Answer from the drawing. Dimensions are ordinates in mm from the lowest x, y and z of the part. A direction names the side the tool comes from. Coordinates: 2 decimals unless noted, no trailing zeros. Write each loop counter-clockwise with the first axis right and the second up, starting at its lowest first coordinate (ties: lowest second). Pieces come first, ordered by that corner, then holes.
(1) The part is cut by section A-A on x = 3. Determine the outline of the cut face in (y, z), plus the area to 3 significant figures.
(2) Which of the six approach directions +Z, -Z, +X, -X, +Y, -Y give full straight-line access (tool end or side, diameter ignored) to the marked faces 4, 5 and 6?
(3) The part is cut by section D-D on y = 5.5. Determine the outline of the cut face in (x, z), plus the area to 3 significant figures.
(4) For a pull along Z with two mould halves and no side action, classify the marked faces 1, 2 and 3 as +Z half, -Z half, draft (parallel to the pull), parting line (faces both ways), or undercut.
(5) The part is cut by section C-C on z = 9. Determine the outline of the cut face in (x, y).
(6) Straight lines are drawn through the part: line 1 (Z direction, x = 3, y = 2.2); line 2 (X direction, y = 1.25, z = 9); line 3 (Y direction, x = 7.2, z = 8). For each, find the intervals that lie inside material, in ascending order.
(7) The part is cut by section B-B on y = 1.5. Determine the outline of the cut face in (x, z), plus the area to 3 significant figures.
(8) Given P1, Ø5, axis at x = 20, z = 3.5, coming from the +Y side (1 decimal); P2, Ø5, axis at x = 21, z = 3, coming from the +Y side; P3, Ø2, axis at y = 4, z = 1.5, coming from the +X side, each flat-ended and moving along its own axis, determine where each tip first touches the part or whether it passes through.
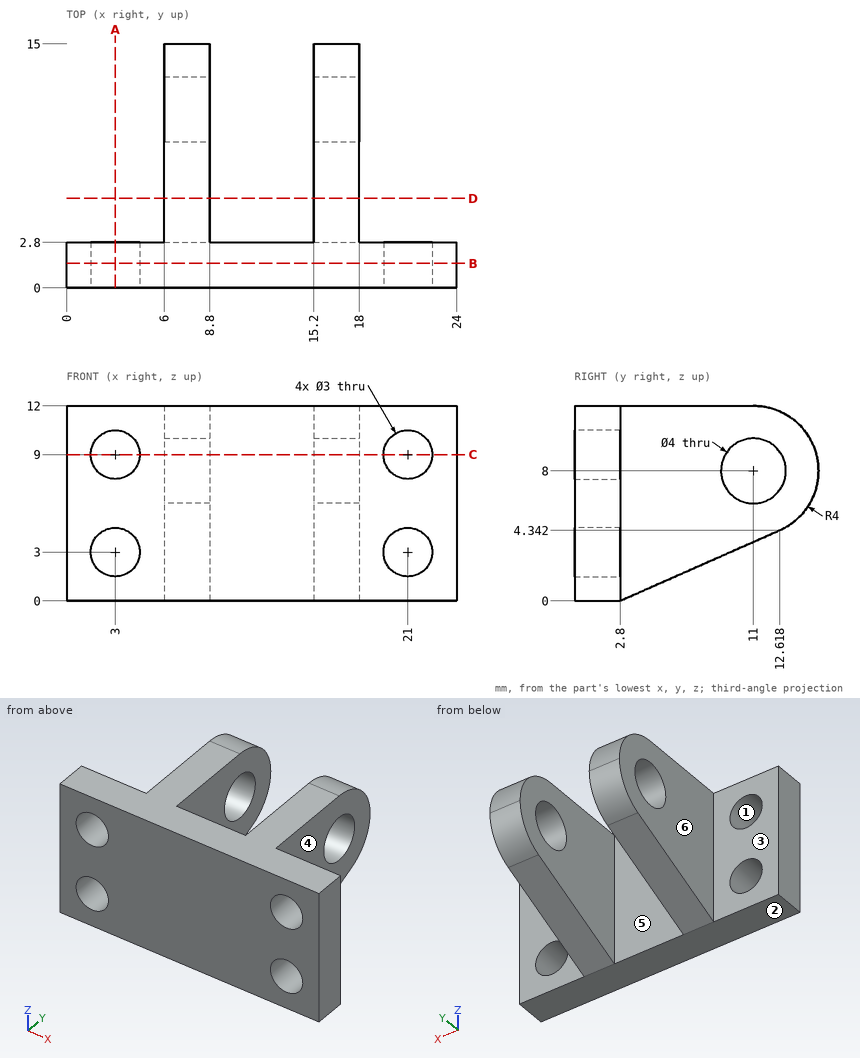
Model answer:
1. outline: (0, 0) - (2.8, 0) - (2.8, 1.5) - (0, 1.5) - close; (0, 4.5) - (2.8, 4.5) - (2.8, 7.5) - (0, 7.5) - close; (0, 10.5) - (2.8, 10.5) - (2.8, 12) - (0, 12) - close
1. area: 16.8 mm2
2. face 4: +Z, -Z, +X, +Y
2. face 5: +Z, -Z, +Y
2. face 6: +Z, -Z, -X, +Y
3. outline: (6, 1.19) - (8.8, 1.19) - (8.8, 12) - (6, 12) - close; (15.2, 1.19) - (18, 1.19) - (18, 12) - (15.2, 12) - close
3. area: 60.5 mm2
4. face 1: undercut
4. face 2: -Z half
4. face 3: draft
5. outline: (0, 0) - (1.5, 0) - (1.5, 2.8) - (0, 2.8) - close; (4.5, 0) - (19.5, 0) - (19.5, 2.8) - (18, 2.8) - (18, 9.27) - (15.2, 9.27) - (15.2, 2.8) - (8.8, 2.8) - (8.8, 9.27) - (6, 9.27) - (6, 2.8) - (4.5, 2.8) - close; (6, 12.73) - (8.8, 12.73) - (8.8, 14.87) - (6, 14.87) - close; (15.2, 12.73) - (18, 12.73) - (18, 14.87) - (15.2, 14.87) - close; (22.5, 0) - (24, 0) - (24, 2.8) - (22.5, 2.8) - close
6. line 1: z = 0 to 1.5, 4.5 to 7.5, 10.5 to 12
6. line 2: x = 0 to 1.5, 4.5 to 19.5, 22.5 to 24
6. line 3: y = 0 to 9, 13 to 15
7. outline: (0, 0) - (24, 0) - (24, 12) - (0, 12) - close; hole circle Ø3 at (3, 3); hole circle Ø3 at (3, 9); hole circle Ø3 at (21, 3); hole circle Ø3 at (21, 9)
7. area: 260 mm2
8. P1: stops at y = 13.6
8. P2: stops at y = 2.8
8. P3: stops at x = 18
